Autodesk Inventor part; units mm, degrees
ref_plane "YZ Plane" through (0, 0, 0) normal (1, 0, 0) x (0, 1, 0)
ref_plane "XZ Plane" through (0, 0, 0) normal (0, 1, 0) x (-1, 0, 0)
ref_plane "XY Plane" through (0, 0, 0) normal (0, 0, 1) x (1, 0, 0)
sketch "Sketch1" plane through (0, 0, 0) normal (0, 0, 1) x (1, 0, 0)
  line L0 (-55.5, 81) -> (55.5, 81)
  line L1 (55.5, 81) -> (55.5, -81)
  line L2 (55.5, -81) -> (-55.5, -81)
  line L3 (-55.5, -81) -> (-55.5, 81)
  point P0 (0, 0)
  point P1 (55.5, 0)
  point P2 (0, -81)
  dimension "d0" = 111
  dimension "d1" = 162
extrude "Extrusion1" add sketch "Sketch1" along normal blind 4
sketch "Sketch2" plane through (-55.5, -81, 0) normal (-1, 0, 0) x (0, 0, 1)
  line L0 (4, 0) -> (4, 162)
  line L1 (0, 121) -> (4, 121)
  line L2 (4, 121) -> (4, 41)
  line L3 (4, 41) -> (0, 41)
  line L4 (0, 41) -> (0, 121)
  line L5 (0, 162) -> (0, 0)
  point P0 (0, 81)
  point P1 (0, 81)
  dimension "d4" = 80
  dimension "d5" = 40
extrude "Extrusion2" add sketch "Sketch2" along normal blind 4
sketch "Sketch3" plane through (-55.5, 81, 0) normal (0, 1, 0) x (1, 0, 0)
  line L0 (111, -4) -> (0, -4)
  line L1 (111, 0) -> (0, 0)
  line L2 (30.5, -4) -> (80.5, -4)
  line L3 (80.5, -4) -> (80.5, 0)
  line L4 (80.5, 0) -> (30.5, 0)
  line L5 (30.5, 0) -> (30.5, -4)
  point P0 (55.5, 0)
  point P1 (80.5, -2)
  point P2 (30.5, -2)
  point P3 (55.5, 0)
  point P4 (30.5, 0)
  dimension "d8" = 50
  dimension "d9" = 25
extrude "Extrusion3" add sketch "Sketch3" along normal blind 4
mirror "Mirror1" about plane through (0, 0, 0) normal (0, 1, 0) of "Extrusion3"
sketch "Sketch4" plane through (55.5, -81, 0) normal (1, 0, 0) x (0, 0, -1)
  line L0 (-4, 0) -> (-4, 162)
  line L1 (0, 0) -> (0, 162)
  line L2 (-4, 0) -> (0, 0)
  line L3 (0, 0) -> (0, 162)
  line L4 (0, 162) -> (-4, 162)
  line L5 (-4, 162) -> (-4, 0)
  point P0 (0, 81)
extrude "Extrusion4" add sketch "Sketch4" along normal blind 4
properties part number "Tapa Superior"
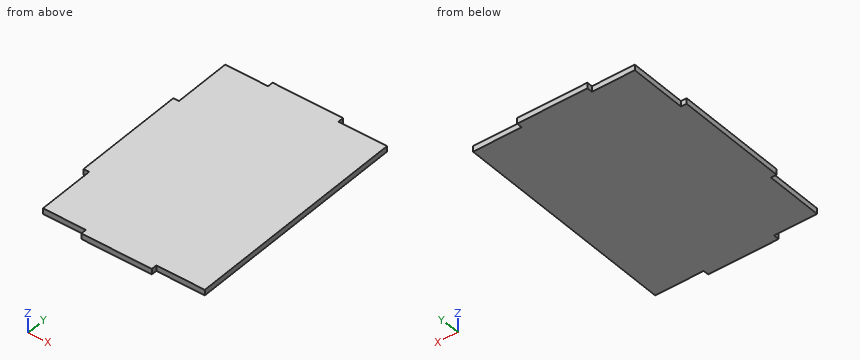
Can you work these out from the model? Positions are in its coordinate system, mm. Round coordinates to 2 decimals unless told otherwise and drop trailing zeros. Order: outer loops, then holes, each group sorted by start corner. A loop starts at its lowest first (then second) coordinate and runs counter-clockwise, first axis right, second up. Notation, with made-up numbers: (81, -4) -> (134, -4) arc R28 cw to (134, 26) -> close; hole circle Ø1 at (14.5, 37.25). An arc over 180 degrees is marked (long way). Return JSON: item names as keys, results as strings. Group by question number.
1. Will these pins go through, and if not, where does the flat tip stop? pin 1 (1.2 mm diameter, centred on x = 37, z = 3, fed in from +Y); pin 2 (1.2 mm diameter, centred on x = 40.5, z = 3, fed in from -Y); pin 3 (2 mm diameter, centred on y = -82.5, z = 1.5, fed in from -X).
2. If we section it at B-B, the plane y = -71.5: Write out the boundary of the cut face in (x, z), then the cut area to 3 significant figures.
3. If we section it at A-A, the plane z = 3.15: Write out the boundary of the cut face in (x, y).
4. I need wall thicknesses on line 1 (X direction, y = 78, z = 3.7); line 2 (Y direction, x = 29, z = 2.2). Which ranges of each line are inside material? Lowest first, please. Write a range as [from, to].
5. If we section it at C-C, the plane x = 42: Write out the boundary of the cut face in (y, z), then the cut area to 3 significant figures.
Output values:
{
 "1": {"pin 1": "y = 81", "pin 2": "y = -81", "pin 3": "x = -25"},
 "2": {"outline": "(-55.5, 0) -> (59.5, 0) -> (59.5, 4) -> (-55.5, 4) -> close", "area": "460 mm²"},
 "3": {"outline": "(-59.5, -40) -> (-55.5, -40) -> (-55.5, -81) -> (-25, -81) -> (-25, -85) -> (25, -85) -> (25, -81) -> (59.5, -81) -> (59.5, 81) -> (25, 81) -> (25, 85) -> (-25, 85) -> (-25, 81) -> (-55.5, 81) -> (-55.5, 40) -> (-59.5, 40) -> close"},
 "4": {"line 1": "[-55.5, 59.5]", "line 2": "[-81, 81]"},
 "5": {"outline": "(-81, 0) -> (81, 0) -> (81, 4) -> (-81, 4) -> close", "area": "648 mm²"}
}
